The figure shows three views and two pictorial views of one solid part (mm, origin at its lowest corner). Answer the questions. A direction names the side the tool comes from. Give positions to 0.01 mm unless a question says otherwise; leave off trailing zeros. Loops run counter-clockwise (first coordinate to the right, second up) from the corner with the lowest first, then second, coordinate; pieces in that order, holes last. Notation, with made-up numbers: (17.5, 35.25) - (51.5, 35.25) arc R17 cw to (51.5, 46.25) - close; hole circle Ø1 at (68, 70.5). An arc over 180 degrees is marked (long way). Write each question's results on one line, items separated by ' | '.
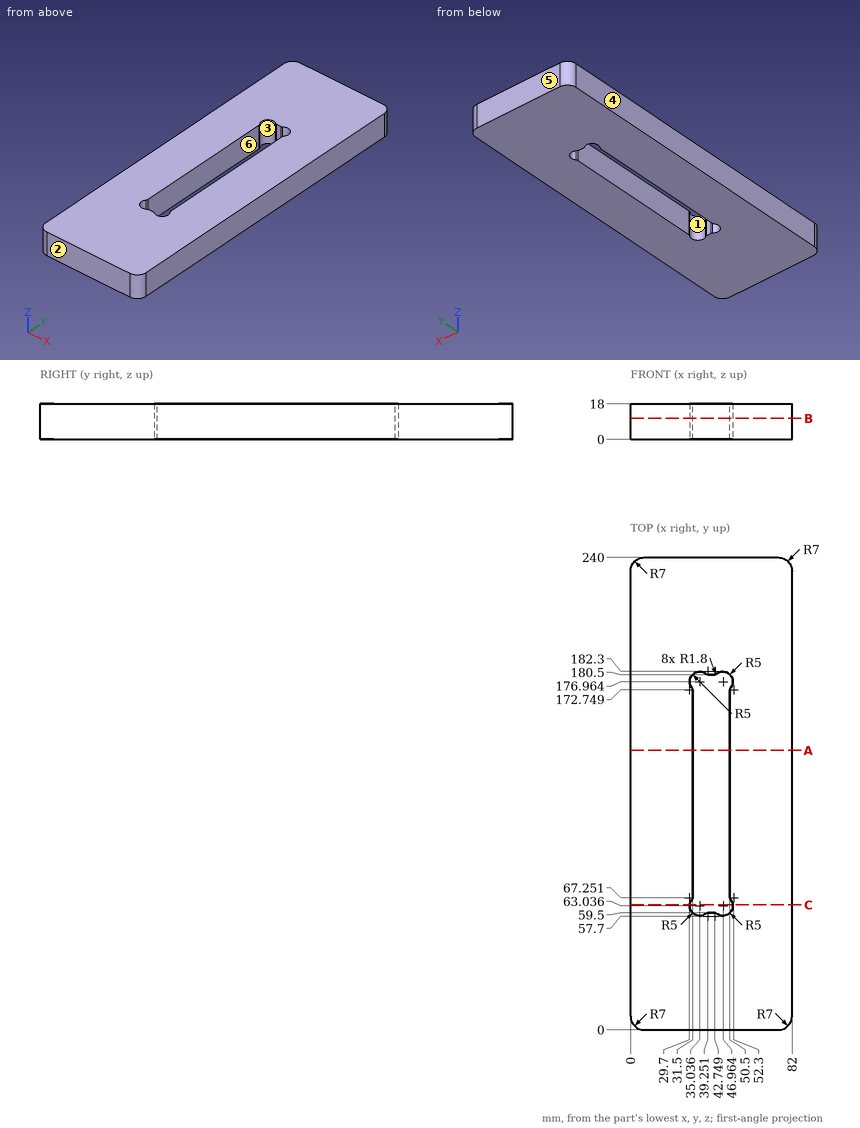
Item 1: A flat-ended cylindrical pin translates along its axis: P1, Ø10, axis at x = 73.5, z = 5.5, coming from the -Y side. Find the tip coordinate at first contact, or state that the pin passes through.
Values found:
P1: stops at y = 0
Item 2: A cutting plane is placed at C-C, the plane y = 63.5. Determine the outline of the cut face in (x, z), plus the area to 3 significant figures.
Values found:
outline: (0, 0) - (30.06, 0) - (30.06, 18) - (0, 18) - close; (51.94, 0) - (82, 0) - (82, 18) - (51.94, 18) - close | area: 1,080 mm²
Item 3: Find the intervals of material crossed by line 1 along Y through (x, z) = (39.5, 15.5); line 2 along X through (y, z) = (63.5, 11.25); line 3 along X through (y, z) = (145, 17.25), in increasing order. Write a range as [from, to].
Values found:
line 1: y = [0, 59.5], [180.5, 240] | line 2: x = [0, 30.06], [51.94, 82] | line 3: x = [0, 31.5], [50.5, 82]
Item 4: A cutting plane is placed at A-A, the plane y = 142. Determine the outline of the cut face in (x, z), plus the area to 3 significant figures.
Values found:
outline: (0, 0) - (31.5, 0) - (31.5, 18) - (0, 18) - close; (50.5, 0) - (82, 0) - (82, 18) - (50.5, 18) - close | area: 1,130 mm²
Item 5: For a pull along Y with two mould halves and no side action, classify the marked faces 1, 2, 3 and 4 as released by +Y, released by -Y, zero draft, split by the parting line, or undercut.
Values found:
face 1: undercut | face 2: released by -Y | face 3: undercut | face 4: zero draft
Item 6: A cutting plane is placed at B-B, the plane z = 10.75. Determine the outline of the cut face in (x, y) (1 decimal), plus the area to 3 significant figures.
Values found:
outline: (0, 7) arc R7 ccw to (7, 0) - (75, 0) arc R7 ccw to (82, 7) - (82, 233) arc R7 ccw to (75, 240) - (7, 240) arc R7 ccw to (0, 233) - close; hole (31.1, 66.1) arc R5 ccw to (38.1, 59.1) arc R1.8 cw to (39.3, 59.5) - (42.7, 59.5) arc R1.8 cw to (43.9, 59.1) arc R5 ccw to (50.9, 66.1) arc R1.8 cw to (50.5, 67.3) - (50.5, 172.7) arc R1.8 cw to (50.9, 173.9) arc R5 ccw to (43.9, 180.9) arc R1.8 cw to (42.7, 180.5) - (39.3, 180.5) arc R1.8 cw to (38.1, 180.9) arc R5 ccw to (31.1, 173.9) arc R1.8 cw to (31.5, 172.7) - (31.5, 67.3) arc R1.8 cw to start | area: 17,300 mm²
Item 7: For the marked faces 5 and 6, determine the directions among +Z, -Z, +X, -X, +Y, -Y from which every point of the face is accessible in a straight line to the end or side of a thin tool.
Values found:
face 5: +Z, -Z, +X, -X, +Y | face 6: +Z, -Z
